Check sheet for the modelled part. Datum: model origin and axes. Units: mm. Give positions to 0.01 mm unless a question says otherwise; leave off trailing zeros. Write each loop counter-clockwise with the first axis right and the second up, starting at its lowest first coordinate (ties: lowest second). Pieces come first, ordered by that corner, then holes. Notation, with made-up numbers: (-27.5, -9) -> (20.5, -9) arc R13 cw to (20.5, 2) -> close; hole circle Ø2 at (67, 66.5). An arc over 180 degrees is marked (long way). Answer as a JSON object with one key per item and string values.
from build123d import *

# Parameters (mm, degrees)
F0_W     = 130
F0_H     = 197
F1_DEPTH = 3
F3_DEPTH = 9.652


with BuildPart() as f1:
    # F0 (on Top) → F1 (new body)
    with BuildSketch(Plane.XY):
        Rectangle(F0_W, F0_H)
    extrude(amount=F1_DEPTH)

    # F2 (on Top) → F3 (cut)
    with BuildSketch(Plane.XY):
        Polygon((6.758312, 0), (6.758312, 17.78), (-3.241688, 17.78), (-3.241688, 0), (-21.021688, 0), (-21.021688, -10.0076), (-3.241688, -10.0076), (-3.241688, -27.7876), (6.765912, -27.7876), (6.765912, -10.0076), (24.545912, -10.0076), (24.545912, 0), align=None)
    extrude(amount=F3_DEPTH, mode=Mode.SUBTRACT)


solid = f1.part
1. Sectioned sample at C-C, the plane z = 2.2. Enter the section's corners in (x, y), plus the area to 3 significant figures.
Determined:
{"outline": "(-65, -98.5) -> (65, -98.5) -> (65, 98.5) -> (-65, 98.5) -> close; hole (-21.02, -10.01) -> (-3.24, -10.01) -> (-3.24, -27.79) -> (6.77, -27.79) -> (6.77, -10.01) -> (24.55, -10.01) -> (24.55, 0) -> (6.76, 0) -> (6.76, 17.78) -> (-3.24, 17.78) -> (-3.24, 0) -> (-21.02, 0) -> close", "area": "24,800 mm^2"}
2. Sectioned sample at A-A, the plane x = -8.5. Enter the section's corners in (y, z), plus the area to 3 significant figures.
Determined:
{"outline": "(-98.5, 0) -> (-10.01, 0) -> (-10.01, 3) -> (-98.5, 3) -> close; (0, 0) -> (98.5, 0) -> (98.5, 3) -> (0, 3) -> close", "area": "561 mm^2"}
3. Sectioned sample at B-B, the plane y = -17. Enter the section's corners in (x, z), plus the area to 3 significant figures.
Determined:
{"outline": "(-65, 0) -> (-3.24, 0) -> (-3.24, 3) -> (-65, 3) -> close; (6.77, 0) -> (65, 0) -> (65, 3) -> (6.77, 3) -> close", "area": "360 mm^2"}
4. Scan lines: L1, parallel to Y at x = 22, z = 2.65; L2, parallel to X at y = -3, z = 2.3; L3, parallel to X at y = -11, z = 1.25. Record each from-to range of solid material in increasing order. Write a range as [from, to].
Determined:
{"L1": "[-98.5, -10.01], [0, 98.5]", "L2": "[-65, -21.02], [24.55, 65]", "L3": "[-65, -3.24], [6.77, 65]"}
